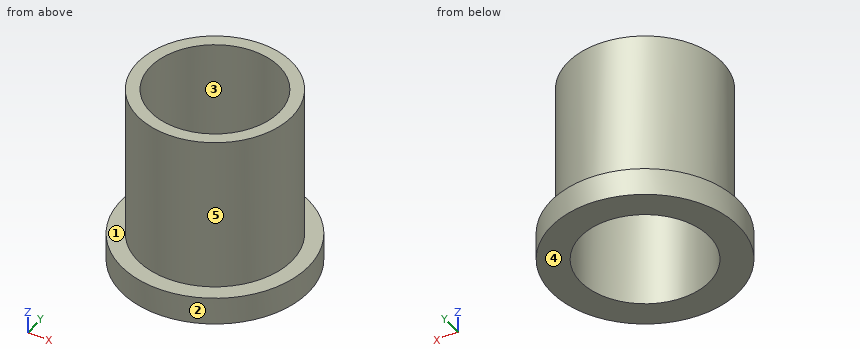
from build123d import *

# Parameters (mm, degrees)
CYLINDER093_R     = 1.5
CYLINDER093_DEPTH = 14
CYLINDER090_R     = 11.7
CYLINDER090_DEPTH = 33
CYLINDER094_R     = 1.5
CYLINDER094_DEPTH = 14
CYLINDER088_R     = 14
CYLINDER088_DEPTH = 33
BOX016_W          = 1
BOX016_H          = 1
BOX016_DEPTH      = 1
CYLINDER084_R     = 17
CYLINDER084_DEPTH = 5


with BuildPart() as obj1:
    # Cylinder093 → Cylinder093 (new body)
    with BuildSketch(Plane(origin=(53.66, 148, -15), x_dir=(1, 0, 0), z_dir=(0, 0, 1))):
        Circle(CYLINDER093_R)
    extrude(amount=CYLINDER093_DEPTH)


with BuildPart() as obj2:
    # Cylinder090 → Cylinder090 (new body)
    with BuildSketch(Plane(origin=(73.66, 148, -10), x_dir=(1, 0, 0), z_dir=(0, 0, 1))):
        Circle(CYLINDER090_R)
    extrude(amount=CYLINDER090_DEPTH)


with BuildPart() as fusion039:
    # Cylinder094 → Cylinder094 (new body)
    with BuildSketch(Plane(origin=(93.66, 148, -14), x_dir=(1, 0, 0), z_dir=(0, 0, 1))):
        Circle(CYLINDER094_R)
    extrude(amount=CYLINDER094_DEPTH)

    # Fusion039: union obj1, obj2
    add(obj1.part)
    add(obj2.part)


with BuildPart() as obj3:
    # Cylinder088 → Cylinder088 (new body)
    with BuildSketch(Plane(origin=(73.66, 148, -10), x_dir=(1, 0, 0), z_dir=(0, 0, 1))):
        Circle(CYLINDER088_R)
    extrude(amount=CYLINDER088_DEPTH)


with BuildPart() as obj4:
    # Box016 → Box016 (new body)
    with BuildSketch(Plane(origin=(63, 136, -8), x_dir=(1, 0, 0), z_dir=(0, 0, 1))):
        with Locations((0.5, 0.5)):
            Rectangle(BOX016_W, BOX016_H)
    extrude(amount=BOX016_DEPTH)


with BuildPart() as obj5:
    # Cylinder084 → Cylinder084 (new body)
    with BuildSketch(Plane(origin=(73.66, 148, -10), x_dir=(1, 0, 0), z_dir=(0, 0, 1))):
        Circle(CYLINDER084_R)
    extrude(amount=CYLINDER084_DEPTH)

    # Fusion038: union obj3, obj4
    add(obj3.part)
    add(obj4.part)

    # Cut010: cut Fusion039
    add(fusion039.part, mode=Mode.SUBTRACT)


with BuildPart() as obj5_1:
    # Cut010 placement: moved
    add(obj5.part.moved(Location((-73.66, -148, -23))))


solid = obj5_1.part
Verification items for the finished model (mm, model axes). Face numbers are marked on the shaded views. A direction names the side the tool comes from. Give positions to 0.01 mm unless a question says otherwise; leave off trailing zeros. Write each loop counter-clockwise with the first axis right and the second up, starting at its lowest first coordinate (ties: lowest second). Pieces come first, ordered by that corner, then holes. Notation, with made-up numbers: M 20,47 L 68,47 A20 ccw 68,74 Z; hole C 62,72.25 d5. An arc over 180 degrees is marked long. Put each result on its own line as item: value. Start each with the question number.
1. Scan lines: line 1 along Y through (x, z) = (0, -22); line 2 along Y through (x, z) = (-0.5, -29.5); line 3 along Z through (x, y) = (-7.5, 14). Record each from-to range of solid material in increasing order. Write a range as [from, to].
2. Draft check along Y on the marked faces 3, 4 and 5. Enter one of: +Y half, -Y half, draft (parallel to the pull), parting line (faces both ways), or undercut.
3. Section check A-A (y = 0). Record the cut outline in (x, z).
4. Section check C-C (z = -23). Record the cut outline in (x, y).
5. Set-up check for the marked faces 1 and 2: record each of +Z, -Z, +X, -X, +Y, -Y from which the full face is reachable in a straight line by a thin tool's end or side.
6. Section check B-B (x = -8.5). Record the cut outline in (y, z), and give its area (3 significant figures).
7. Section check D-D (y = -12.5). Record the cut outline in (x, z).
8. Go/stop test with flat-tipped pins: pin 1 Ø3 at (x, z) = (-12.5, -20.5) entering from -Y; pin 2 Ø8 at (y, z) = (5, -7.5) entering from +X; pin 3 Ø2 at (x, z) = (-4.5, -16.5) entering from -Y. Record where each tip stops, or that it passes through.
Answer list:
1. line 1: [-14, -11.7], [11.7, 14]
1. line 2: [-16.99, -11.69], [11.69, 16.99]
1. line 3: [-33, -28]
2. face 3: undercut
2. face 4: draft
2. face 5: parting line
3. outline: M -17,-33 L -11.7,-33 L -11.7,0 L -14,0 L -14,-28 L -17,-28 Z; M 11.7,-33 L 17,-33 L 17,-28 L 14,-28 L 14,0 L 11.7,0 Z
4. outline: C 0,0 d28; hole C 0,0 d23.4
5. face 1: +Z
5. face 2: +Z, -Z
6. outline: M -14.72,-33 L -8.04,-33 L -8.04,0 L -11.12,0 L -11.12,-28 L -14.72,-28 Z; M 8.04,-33 L 14.72,-33 L 14.72,-28 L 11.12,-28 L 11.12,0 L 8.04,0 Z
6. area: 240 mm2
7. outline: M -11.52,-33 L 11.52,-33 L 11.52,-28 L 6.3,-28 L 6.3,0 L -6.3,0 L -6.3,-28 L -11.52,-28 Z
8. pin 1: y = -8.66
8. pin 2: x = 13.96
8. pin 3: y = -13.56
